```python
from build123d import *

# Parameters (mm, degrees)
ESQUISSE1_W        = 40
ESQUISSE1_H        = 50
ESQUISSE1_R        = 2
BOSS_EXTRU_1_DEPTH = 2
ESQUISSE4_W        = 40
ESQUISSE4_H        = 50
ESQUISSE4_R        = 2
BOSS_EXTRU_3_DEPTH = 2


with BuildPart() as part:
    # Esquisse1 → Boss.-Extru.1 (new body)
    with BuildSketch(Plane(origin=(0, 0, 0), x_dir=(1, 0, 0), z_dir=(0, 1, 0))):
        with Locations((0, 3)):
            Rectangle(ESQUISSE1_W, ESQUISSE1_H)
        with Locations(Location((0, 0, 0), (0, 0, 270))):
            Circle(ESQUISSE1_R, mode=Mode.SUBTRACT)
        with Locations(Location((-12, -14, 0), (0, 0, 270))):
            Circle(ESQUISSE1_R, mode=Mode.SUBTRACT)
        with Locations(Location((-12, 16, 0), (0, 0, 270))):
            Circle(ESQUISSE1_R, mode=Mode.SUBTRACT)
        with Locations(Location((12, 16, 0), (0, 0, 270))):
            Circle(ESQUISSE1_R, mode=Mode.SUBTRACT)
        with Locations(Location((12, -14, 0), (0, 0, 270))):
            Circle(ESQUISSE1_R, mode=Mode.SUBTRACT)
    extrude(amount=BOSS_EXTRU_1_DEPTH)

    # Esquisse4 → Boss.-Extru.3 (add)
    with BuildSketch(Plane(origin=(0, 0, -28), x_dir=(-1, 0, 0), z_dir=(0, 0, -1))):
        with Locations((0, 25)):
            Rectangle(ESQUISSE4_W, ESQUISSE4_H)
        with Locations((0, 28)):
            Circle(ESQUISSE4_R, mode=Mode.SUBTRACT)
        with Locations((12, 42)):
            Circle(ESQUISSE4_R, mode=Mode.SUBTRACT)
        with Locations((-12, 42)):
            Circle(ESQUISSE4_R, mode=Mode.SUBTRACT)
        with Locations((-12, 14)):
            Circle(ESQUISSE4_R, mode=Mode.SUBTRACT)
        with Locations((12, 14)):
            Circle(ESQUISSE4_R, mode=Mode.SUBTRACT)
    extrude(amount=-BOSS_EXTRU_3_DEPTH)


solid = part.part
```
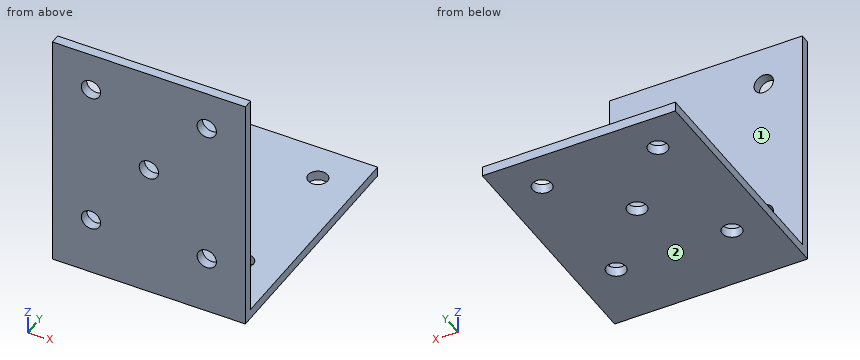
Geometry check sheet. Reference: the model listing, model coordinates, mm. Face numbers are marked on the shaded views. A direction names the side the tool comes from. Round coordinates to 2 decimals unless told otherwise and drop trailing zeros. Loops run counter-clockwise (first coordinate to the right, second up) from the corner with the lowest first, then second, coordinate; pieces in that order, holes last. Notation, with made-up numbers: (-22, -16) -> (33, -16) arc R33 cw to (33, 17) -> close; hole circle Ø3 at (23, 26.5). An arc over 180 degrees is marked (long way). Use a Markdown table: item, result.
(1) Sectioned sample at D-D (y = 28). Enter the section's corners in (x, z).
Calculated:
| item | result |
|---|---|
| outline | (-20, -28) -> (-2, -28) -> (-2, -26) -> (-20, -26) -> close; (2, -28) -> (20, -28) -> (20, -26) -> (2, -26) -> close |
(2) Scan lines: probe 1 along X at (y, z) = (1, -16); probe 2 along Y at (x, z) = (-12, -27); probe 3 along X at (y, z) = (1.2, 0). Record each from-to range of solid material in increasing order.
Calculated:
| item | result |
|---|---|
| probe 1 | -20 to -14, -10 to 10, 14 to 20 |
| probe 2 | 0 to 12, 16 to 40, 44 to 50 |
| probe 3 | -20 to -2, 2 to 20 |
(3) Go/stop test with flat-tipped pins: P1, Ø3.5, axis at x = 12, z = -16, coming from the +Y side; P2, Ø12, axis at y = 31, z = -22, coming from the +X side; P3, Ø6.5, axis at x = -12, y = 42, coming from the +Z side; P4, Ø6.5, axis at x = -12, z = -16, coming from the +Y side. Record where each tip stops, or that it passes through.
Calculated:
| item | result |
|---|---|
| P1 | through |
| P2 | x = 20 |
| P3 | z = -26 |
| P4 | y = 2 |
(4) Sectioned sample at B-B (y = 14). Enter the section's corners in (x, z).
Calculated:
| item | result |
|---|---|
| outline | (-20, -28) -> (-14, -28) -> (-14, -26) -> (-20, -26) -> close; (-10, -28) -> (10, -28) -> (10, -26) -> (-10, -26) -> close; (14, -28) -> (20, -28) -> (20, -26) -> (14, -26) -> close |
(5) Sectioned sample at C-C (z = 0). Enter the section's corners in (x, y).
Calculated:
| item | result |
|---|---|
| outline | (-20, 0) -> (-2, 0) -> (-2, 2) -> (-20, 2) -> close; (2, 0) -> (20, 0) -> (20, 2) -> (2, 2) -> close |
(6) Set-up check for the marked faces 1 and 2: record each of +Z, -Z, +X, -X, +Y, -Y from which the full face is reachable in a straight line by a thin tool's end or side.
Calculated:
| item | result |
|---|---|
| face 1 | +Z, +X, -X, +Y |
| face 2 | -Z, +X, -X, +Y, -Y |
(7) Sectioned sample at A-A (x = 0). Enter the section's corners in (y, z), then the cut area to 3 significant figures.
Calculated:
| item | result |
|---|---|
| outline | (0, -28) -> (26, -28) -> (26, -26) -> (2, -26) -> (2, -2) -> (0, -2) -> close; (0, 2) -> (2, 2) -> (2, 22) -> (0, 22) -> close; (30, -28) -> (50, -28) -> (50, -26) -> (30, -26) -> close |
| area | 180 mm² |
